Build history of the part. All positions in model axes, mm. Coordinates: 2 decimals unless noted, no trailing zeros. Loops run counter-clockwise (first coordinate to the right, second up) from the corner with the lowest first, then second, coordinate; pieces in that order, holes last.
(1) Slice it at A-A (y = 21.73). Give the cut face in (x, z), and give its area (3 significant figures).
(2) Slice it at B-B (x = 11.5). Give the cut face in (y, z), and give its area (3 significant figures).
(3) Slice it at C-C (z = 1). Give the cut face in (x, y).
(4) Slice it at D-D (y = 13.5). Give the cut face in (x, z).
(5) Flat gauge pins, fed straight in: P1, Ø1.8, axis at x = 28.5, y = -8.6, coming from the +Z side; P2, Ø1, axis at y = 22, z = 1.5, coming from the -X side. Where does each tip first touch, or does it go through?
(6) Wall check: L1, parallel to X at y = -9, z = 0.4; L2, parallel to X at y = -11, z = 1.35; L3, parallel to Y at x = 28.5, z = 1.15. Give the ranges that are in metal, low to high.
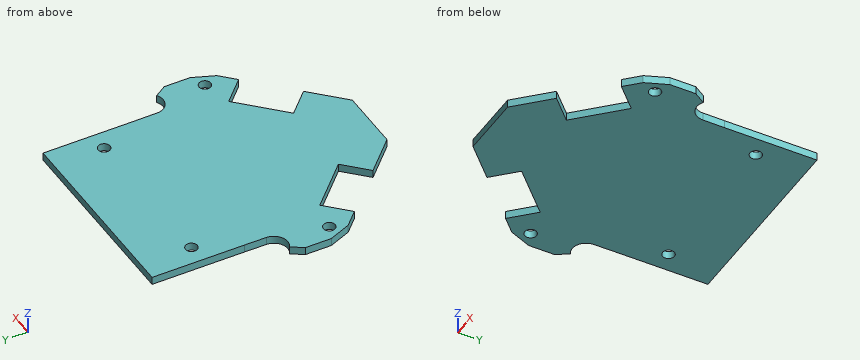
from build123d import *

# Parameters (mm, degrees)
EXTRUDE1_DEPTH  = 2
SKETCH4_R       = 1.5
EXTRUDE3_DEPTH  = 2
EXTRUDE5_DEPTH  = 2
FILLET2_R       = 3
SKETCH7_R       = 1.5
EXTRUDE6_DEPTH  = 2
EXTRUDE7_DEPTH  = 2
EXTRUDE8_DEPTH  = 2
EXTRUDE9_DEPTH  = 2
EXTRUDE10_DEPTH = 2
EXTRUDE11_DEPTH = 2
SKETCH13_W      = 52.444820885
SKETCH13_H      = 24.426279397
EXTRUDE12_DEPTH = 2
SKETCH14_R      = 1.5
EXTRUDE13_DEPTH = 2
EXTRUDE14_DEPTH = 2
EXTRUDE15_DEPTH = 2
SKETCH17_W      = 50
SKETCH17_H      = 4
EXTRUDE17_DEPTH = 2


with BuildPart() as part:
    # Sketch1 → Extrude1 (new body)
    with BuildSketch(Plane.XY):
        Polygon((-15, 13.5), (-15, 38.5), (15, 38.5), (15, 13.5), (26.811651575, -4.688348425), (15, -16.5), (15, -26.5), (7.928932188, -33.571067812), (7.928932188, -52.571067812), (-7.928932188, -52.571067812), (-7.928932188, -33.571067812), (-15, -26.5), (-15, -16.5), (-26.811651575, -4.688348425), align=None)
    extrude(amount=EXTRUDE1_DEPTH)

    # Sketch4 → Extrude3 (add)
    with BuildSketch(Plane.XY.offset(2)):
        Polygon((-26.811651575, -4.688348425), (-32.363678884, -6.963209468), (-30.088817841, -12.515236776), (-22.212122569, -9.287877431), align=None)
        with Locations((-28.5, -8.6)):
            Circle(SKETCH4_R, mode=Mode.SUBTRACT)
    extrude3 = extrude(amount=-EXTRUDE3_DEPTH)

    # Mirror1: Extrude3 across plane
    add(extrude3.mirror(Plane(origin=(0, 0, 0), x_dir=(0, 0, 1), z_dir=(1, 0, 0))))

    # Sketch6 → Extrude5 (add)
    with BuildSketch(Plane.XY.offset(2)):
        Polygon((0, -44.571067812), (-7.928932188, -44.571067812), (-18, -54.642135624), (18, -54.642135624), (7.928932188, -44.571067812), align=None)
    extrude(amount=-EXTRUDE5_DEPTH)

    # Fillet2
    fillet2_edges = [part.edges().sort_by_distance(p)[0] for p in [
        (18, -54.642135624, 1),
        (-18, -54.642135624, 1),
    ]]
    fillet(fillet2_edges, radius=FILLET2_R)

    # Sketch7 → Extrude6 (cut)
    with BuildSketch(Plane.XY.offset(2)):
        with Locations((-11, -52.002135624)):
            Circle(SKETCH7_R)
    extrude6 = extrude(amount=-EXTRUDE6_DEPTH, mode=Mode.SUBTRACT)

    # Mirror4: Extrude6 across plane
    add(extrude6.mirror(Plane(origin=(0, 0, 0), x_dir=(0, 0, 1), z_dir=(1, 0, 0))), mode=Mode.SUBTRACT)

    # Sketch8 → Extrude7 (add)
    with BuildSketch(Plane.XY.offset(2)):
        Polygon((-26.811651575, -4.688348425), (-32.363678884, -6.963209468), (-32.363678884, -0.385171544), (-15, 26.352549211), (-15, 13.5), align=None)
    extrude7 = extrude(amount=-EXTRUDE7_DEPTH)

    # Sketch9 → Extrude8 (add)
    with BuildSketch(Plane.XY.offset(2)):
        Polygon((-22.212122569, -9.287877431), (-25.22165278, -10.520987907), (-15, -20.742640687), (-15, -16.5), align=None)
    extrude8 = extrude(amount=-EXTRUDE8_DEPTH)

    # Sketch10 → Extrude9 (add)
    with BuildSketch(Plane.XY.offset(2)):
        Polygon((-25.22165278, -10.520987907), (-30.088817841, -12.515236776), (-23.702612277, -18.90144234), (-20.271905312, -15.470735375), align=None)
    extrude9 = extrude(amount=-EXTRUDE9_DEPTH)

    # Sketch11 → Extrude10 (add)
    with BuildSketch(Plane.XY.offset(2)):
        Polygon((-15.322157844, -20.420482843), (-18.752864809, -23.851189808), (-7.928932188, -34.675122429), (-7.928932188, -33.571067812), (-15, -26.5), (-15, -20.742640687), align=None)
    extrude10 = extrude(amount=-EXTRUDE10_DEPTH)

    # Sketch12 → Extrude11 (add)
    with BuildSketch(Plane.XY.offset(2)):
        Polygon((-25, 10.953899573), (-25, 38.5), (-15, 38.5), (-15, 26.352549211), align=None)
    extrude11 = extrude(amount=-EXTRUDE11_DEPTH)

    # Mirror5: Extrude7, Extrude8, Extrude9, Extrude10 across plane
    add(extrude7.mirror(Plane(origin=(0, 0, 0), x_dir=(0, 0, 1), z_dir=(1, 0, 0))))
    add(extrude8.mirror(Plane(origin=(0, 0, 0), x_dir=(0, 0, 1), z_dir=(1, 0, 0))))
    add(extrude9.mirror(Plane(origin=(0, 0, 0), x_dir=(0, 0, 1), z_dir=(1, 0, 0))))
    add(extrude10.mirror(Plane(origin=(0, 0, 0), x_dir=(0, 0, 1), z_dir=(1, 0, 0))))

    # Mirror6: Extrude11 across plane
    add(extrude11.mirror(Plane(origin=(0, 0, 0), x_dir=(0, 0, 1), z_dir=(1, 0, 0))))

    # Sketch13 → Extrude12 (cut)
    with BuildSketch(Plane(origin=(0, 0, 0), x_dir=(-1, 0, 0), z_dir=(0, 0, -1))):
        with Locations((1.088066824, -46.888262128)):
            Rectangle(SKETCH13_W, SKETCH13_H)
    extrude(amount=-EXTRUDE12_DEPTH, mode=Mode.SUBTRACT)

    # Sketch14 → Extrude13 (cut)
    with BuildSketch(Plane.XY.offset(2)):
        with Locations((-20, 21.73)):
            Circle(SKETCH14_R)
        with Locations((20, 21.73)):
            Circle(SKETCH14_R)
    extrude(amount=-EXTRUDE13_DEPTH, mode=Mode.SUBTRACT)

    # Sketch15 → Extrude14 (cut)
    with BuildSketch(Plane(origin=(0, 0, 0), x_dir=(-1, 0, 0), z_dir=(0, 0, -1))):
        Polygon((26.531039402, -16.073015215), (20.874185152, -10.416160966), (10.267583435, -21.022762684), (15.924437684, -26.679616933), align=None)
        Polygon((-26.531039402, -16.073015215), (-20.874185152, -10.416160966), (-10.267583435, -21.022762684), (-15.924437684, -26.679616933), align=None)
    extrude(amount=-EXTRUDE14_DEPTH, mode=Mode.SUBTRACT)

    # Sketch16 → Extrude15 (cut)
    with BuildSketch(Plane(origin=(0, 0, 0), x_dir=(-1, 0, 0), z_dir=(0, 0, -1))):
        with BuildLine():
            Line((-25, 10.953899573), (-25.040153728, 5.502540882))
            ThreePointArc((-25.040153728, 5.502540882), (-26.870098067, 2.426680987), (-30.44639035, 2.567193894))
            Line((-30.44639035, 2.567193894), (-25, 10.953899573))
        make_face()
        with BuildLine():
            Line((25, 10.953899573), (25.040153728, 5.502540882))
            ThreePointArc((25.040153728, 5.502540882), (26.870098067, 2.426680987), (30.44639035, 2.567193894))
            Line((30.44639035, 2.567193894), (25, 10.953899573))
        make_face()
    extrude(amount=-EXTRUDE15_DEPTH, mode=Mode.SUBTRACT)

    # Sketch17 → Extrude17 (cut)
    with BuildSketch(Plane(origin=(0, 0, 0), x_dir=(-1, 0, 0), z_dir=(0, 0, -1))):
        with Locations((0, 36.5)):
            Rectangle(SKETCH17_W, SKETCH17_H)
    extrude(amount=-EXTRUDE17_DEPTH, mode=Mode.SUBTRACT)


solid = part.part
Response values:
1. outline: (-25, 0) - (-21.5, 0) - (-21.5, 2) - (-25, 2) - close; (-18.5, 0) - (18.5, 0) - (18.5, 2) - (-18.5, 2) - close; (21.5, 0) - (25, 0) - (25, 2) - (21.5, 2) - close
1. area: 88.0 mm2
2. outline: (-31.1, 0) - (-22.26, 0) - (-22.26, 2) - (-31.1, 2) - close; (-19.79, 0) - (34.5, 0) - (34.5, 2) - (-19.79, 2) - close
2. area: 126 mm2
3. outline: (-32.36, -6.96) - (-30.09, -12.52) - (-26.53, -16.07) - (-20.87, -10.42) - (-10.27, -21.02) - (-15.92, -26.68) - (-7.93, -34.68) - (7.93, -34.68) - (15.92, -26.68) - (10.27, -21.02) - (20.87, -10.42) - (26.53, -16.07) - (30.09, -12.52) - (32.36, -6.96) - (32.36, -0.39) - (30.45, 2.57) arc R3.5 cw to (25.04, 5.5) - (25, 10.95) - (25, 34.5) - (-25, 34.5) - (-25, 10.95) - (-25.04, 5.5) arc R3.5 cw to (-30.45, 2.57) - (-32.36, -0.39) - close; hole circle Ø3 at (-28.5, -8.6); hole circle Ø3 at (-20, 21.73); hole circle Ø3 at (20, 21.73); hole circle Ø3 at (28.5, -8.6)
4. outline: (-25, 0) - (25, 0) - (25, 2) - (-25, 2) - close
5. P1: passes through
5. P2: stops at x = -25
6. L1: x = -31.53 to -29.95, -27.05 to 27.05, 29.95 to 31.53
6. L2: x = -30.71 to -21.46, -20.29 to 20.29, 21.46 to 30.71
6. L3: y = -14.1 to -10.1, -7.1 to 2
